```python
from build123d import *

# Parameters (mm, degrees)
SKETCH2_R           = 16
BOSS_EXTRUDE1_DEPTH = 3
SKETCH3_R           = 6
SKETCH3_R_2         = 2
CUT_EXTRUDE1_DEPTH  = 3
BOSS_EXTRUDE2_START = 10
SKETCH4_R           = 9
SKETCH4_R_2         = 6
BOSS_EXTRUDE2_DEPTH = 10
SKETCH5_R           = 1.6
CUT_EXTRUDE2_DEPTH  = 10


with BuildPart() as part:
    # Sketch2 → Boss-Extrude1 (new body)
    with BuildSketch(Plane(origin=(0, 0, 0), x_dir=(1, 0, 0), z_dir=(0, 1, 0))):
        with Locations(Location((0, 0, 0), (0, 0, 270))):
            Circle(SKETCH2_R)
    extrude(amount=BOSS_EXTRUDE1_DEPTH)

    # Sketch3 → Cut-Extrude1 (cut)
    with BuildSketch(Plane(origin=(0, 3, 0), x_dir=(1, 0, 0), z_dir=(0, 1, 0))):
        with Locations(Location((0, 0, 0), (0, 0, 270))):
            Circle(SKETCH3_R)
        with Locations(Location((-9.192388155, 9.192388155, 0), (0, 0, 270))):
            Circle(SKETCH3_R_2)
        with Locations(Location((9.192388155, 9.192388155, 0), (0, 0, 270))):
            Circle(SKETCH3_R_2)
        with Locations(Location((9.192388155, -9.192388155, 0), (0, 0, 270))):
            Circle(SKETCH3_R_2)
        with Locations(Location((-9.192388155, -9.192388155, 0), (0, 0, 270))):
            Circle(SKETCH3_R_2)
    extrude(amount=-CUT_EXTRUDE1_DEPTH, mode=Mode.SUBTRACT)

    # Sketch4 → Boss-Extrude2 (add)
    with BuildSketch(Plane(origin=(0, 3, 0), x_dir=(1, 0, 0), z_dir=(0, 1, 0)).offset(BOSS_EXTRUDE2_START)):
        with Locations(Location((0, 0, 0), (0, 0, 270))):
            Circle(SKETCH4_R)
        with Locations(Location((0, 0, 0), (0, 0, 270))):
            Circle(SKETCH4_R_2, mode=Mode.SUBTRACT)
    extrude(amount=-BOSS_EXTRUDE2_DEPTH)

    # Sketch5 → Cut-Extrude2 (cut, symmetric)
    with BuildSketch(Plane.XY):
        with Locations(Location((0, 8.4, 0), (0, 0, 270.000000001))):
            Circle(SKETCH5_R)
    extrude(amount=CUT_EXTRUDE2_DEPTH, both=True, mode=Mode.SUBTRACT)


solid = part.part
```
Design review of the part built by this model. Coordinates are the model's own, in mm. Coordinates: 2 decimals unless noted, no trailing zeros. Loops run counter-clockwise (first coordinate to the right, second up) from the corner with the lowest first, then second, coordinate; pieces in that order, holes last.
Q1. We need section B-B on z = 0. State the section outline as (x, y) points.
Reported:
outline: (-16, 0) - (-6, 0) - (-6, 13) - (-9, 13) - (-9, 3) - (-16, 3) - close; (6, 0) - (16, 0) - (16, 3) - (9, 3) - (9, 13) - (6, 13) - close
Q2. For pin 1 (3.5 mm diameter, centred on x = 0, y = 8.4, fed in from -Z); pin 2 (6 mm diameter, centred on y = 7.5, z = -7.5, fed in from -X); pin 3 (6 mm diameter, centred on x = -7.5, y = 9.5, fed in from +Z), all flat-tipped, find the tip position at first contact; note any pin that passes through.
Reported:
pin 1: stops at z = -9
pin 2: stops at x = -7.79
pin 3: stops at z = 7.79
Q3. We need section D-D on y = 2. State the section outline as (x, z) points.
Reported:
outline: circle Ø32 at (0, 0); hole circle Ø4 at (-9.19, -9.19); hole circle Ø4 at (-9.19, 9.19); hole circle Ø12 at (0, 0); hole circle Ø4 at (9.19, -9.19); hole circle Ø4 at (9.19, 9.19)
Q4. The part is to be moulded in two halves that separate along Z. For faces 1 (the face through (8, 1.5, -10.8)), 2 (the face through (2.703, 8.07, 8.584)), 3 (the face through (-7, 3, 7)), say which applies: +Z half, -Z half, draft (parallel to the pull), parting line (faces both ways), or undercut.
Reported:
face 1: undercut
face 2: parting line
face 3: draft
Q5. We need section C-C on y = 8.4. State the section outline as (x, z) points, and give its area (3 significant figures).
Reported:
outline: (-1.6, -8.86) - (-1.6, -5.78) arc R6 cw to (-1.6, 5.78) - (-1.6, 8.86) arc R9 ccw to start; (1.6, -8.86) arc R9 ccw to (1.6, 8.86) - (1.6, 5.78) arc R6 cw to (1.6, -5.78) - close
area: 122 mm2
Q6. We need section A-A on x = 0. State the section outline as (y, z) points.
Reported:
outline: (0, -16) - (3, -16) - (3, -9) - (6.8, -9) - (6.8, -6) - (0, -6) - close; (0, 6) - (6.8, 6) - (6.8, 9) - (3, 9) - (3, 16) - (0, 16) - close; (10, -9) - (13, -9) - (13, -6) - (10, -6) - close; (10, 6) - (13, 6) - (13, 9) - (10, 9) - close
Q7. To check wall thickness, follow line 1 (X direction, y = 7.25, z = 0); line 2 (Y direction, x = 8.5, z = -4.5); line 3 (X direction, y = 1.75, z = -9). State the ranges of each line that lie inside material, in increasing order.
Reported:
line 1: x = -9 to -6, 6 to 9
line 2: y = 0 to 3
line 3: x = -13.23 to -11.18, -7.2 to 7.2, 11.18 to 13.23
